Here's how the part is built. I have some questions about the finished solid (model axes, mm). A direction names the side the tool comes from. Give positions to 0.01 mm unless a question says otherwise; leave off trailing zeros. Write each loop counter-clockwise with the first axis right and the second up, starting at its lowest first coordinate (ties: lowest second). Pieces come first, ordered by that corner, then holes. Notation, with made-up numbers: (67.5, 85) - (79.5, 85) arc R17 cw to (79.5, 103) - close; hole circle Ø8 at (35.5, -38). An arc over 180 degrees is marked (long way). One line per item, written item: value. Start each with the question number.
1) Please list where these lines run through material, in increasing order: L1, parallel to X at y = 5, z = 0; L2, parallel to X at y = 14.5, z = -3; L3, parallel to Y at x = 2, z = 0. Write a range as [from, to].
2) Imagine slicing it at A-A on z = 0. Write out the boundary of the cut face in (x, y), plus the area to 3 significant figures.
3) We'd pull the mould along X, two halves only. Please class faces 1 (the flat face through (1, 4.5, 4.4)), 2 (the conical face through (0.51, -14.79, -10.76)), 3 (the conical face through (0.507, 1.163, -18.25)), 4 (the flat face through (0.014, 16.632, -0.983)): +X half, -X half, draft (parallel to the pull), parting line (faces both ways), or undercut.
4) I'm going to push flat-ended pins straight in: P1, Ø5, axis at x = 4, z = 6, coming from the +Y side; P2, Ø0.6, axis at x = 0, z = 0.5, coming from the -Y side; P3, Ø5, axis at x = 9, y = 5.5, coming from the +Z side. Where does each tip first touch, or does it pass through?
5) On a 3-axis mill with a long thin cutter (end or side, diameter ignored), from which of +Z, -Z, +X, -X, +Y, -Y can I reach the whole of each face in a straight line? I mean faces 5 (the conical face through (0.51, -3.41, -17.97)), 6 (the conical face through (-0.493, 13.331, -12.498)), 7 (the flat face through (0.01, 2.02, -16.49)). Say none if no direction works.
6) Imagine slicing it at C-C on x = 5.5. Write out the boundary of the cut face in (y, z), plus the area to 3 significant figures.
7) Imagine slicing it at B-B on x = 2.25. Write out the boundary of the cut face in (y, z), plus the area to 3 significant figures.
from build123d import *

# Parameters (mm, degrees)
SKETCH2_R           = 18.78
SKETCH2_R_2         = 4.05
BOSS_EXTRUDE1_DEPTH = 1
SKETCH9_R           = 6.05
SKETCH9_R_2         = 4.05
BOSS_EXTRUDE2_DEPTH = 10
SKETCH10_R          = 1.25
CUT_EXTRUDE1_DEPTH  = 10
CUT_EXTRUDE3_DEPTH  = 10
CIRPATTERN1_COUNT   = 25


with BuildPart() as part:
    # Sketch2 → Boss-Extrude1 (new, symmetric)
    with BuildSketch(Plane(origin=(0, 0, 0), x_dir=(0, 0, -1), z_dir=(1, 0, 0))):
        Circle(SKETCH2_R)
        Circle(SKETCH2_R_2, mode=Mode.SUBTRACT)
    extrude(amount=BOSS_EXTRUDE1_DEPTH, both=True)

    # Sketch9 → Boss-Extrude2 (add)
    with BuildSketch(Plane(origin=(1, 0, 0), x_dir=(0, 0, -1), z_dir=(1, 0, 0))):
        Circle(SKETCH9_R)
        Circle(SKETCH9_R_2, mode=Mode.SUBTRACT)
    extrude(amount=BOSS_EXTRUDE2_DEPTH)

    # Sketch5 → Cut-Revolve1 (revolve, cut)
    with BuildSketch(Plane(origin=(0, 0, 0), x_dir=(1, 0, 0), z_dir=(0, 1, 0)), mode=Mode.PRIVATE) as cut_revolve1_sk:
        Polygon((-1, -18.78), (0, -17.78), (1, -18.78), align=None)
    revolve(cut_revolve1_sk.sketch.rotate(Axis((11, 0, 0), (-1, 0, 0)), 180), axis=Axis((11, 0, 0), (-1, 0, 0)), mode=Mode.SUBTRACT)

    # Sketch10 → Cut-Extrude1 (cut, symmetric)
    with BuildSketch(Plane(origin=(0, 0, 0), x_dir=(1, 0, 0), z_dir=(0, 1, 0))):
        with Locations(Location((6, 0, 0), (0, 0, 270))):
            Circle(SKETCH10_R)
    extrude(amount=CUT_EXTRUDE1_DEPTH, both=True, mode=Mode.SUBTRACT)

    # Sketch12 → Cut-Extrude3 (cut, symmetric)
    with BuildSketch(Plane(origin=(1, 0, 0), x_dir=(0, 0, -1), z_dir=(1, 0, 0))):
        with BuildLine():
            ThreePointArc((-1.25, -18.738353716), (0, -18.78), (1.25, -18.738353716))
            Line((1.25, -18.738353716), (1.016521645, -15.238353716))
            Line((1.016521645, -15.238353716), (-1.016521645, -15.238353716))
            Line((-1.016521645, -15.238353716), (-1.25, -18.738353716))
        make_face()
    cut_extrude3 = extrude(amount=CUT_EXTRUDE3_DEPTH, both=True, mode=Mode.SUBTRACT)

    # CirPattern1: Cut-Extrude3 ×25 about axis
    cirpattern1_axis = Axis((0, 0, 0), (1, 0, 0))
    for i in range(1, CIRPATTERN1_COUNT):
        add(cut_extrude3.rotate(cirpattern1_axis, i * 360 / CIRPATTERN1_COUNT), mode=Mode.SUBTRACT)


solid = part.part
Numbers:
1. L1: [-1, 4.75], [7.25, 11]
1. L2: [-1, 1]
1. L3: [-6.05, -4.05], [4.05, 6.05]
2. outline: (-1, -15.24) - (1, -15.24) - (1, -6.05) - (4.75, -6.05) - (4.75, -4.05) - (-1, -4.05) - close; (-1, 4.05) - (4.75, 4.05) - (4.75, 6.05) - (1, 6.05) - (1, 18.78) - (0, 17.78) - (-1, 18.78) - close; (7.25, -6.05) - (11, -6.05) - (11, -4.05) - (7.25, -4.05) - close; (7.25, 4.05) - (11, 4.05) - (11, 6.05) - (7.25, 6.05) - close
2. area: 80.8 mm^2
3. face 1: +X half
3. face 2: undercut
3. face 3: undercut
3. face 4: draft
4. P1: y = 4.93
4. P2: y = -15.24
4. P3: z = 5.25
5. face 5: -Z, -Y
5. face 6: -Z, +Y
5. face 7: +X, -X
6. outline: (-5.94, -1.15) arc R6.05 ccw to (5.94, -1.15) - (3.88, -1.15) arc R4.05 cw to (-3.88, -1.15) - close; (-5.94, 1.15) - (-3.88, 1.15) arc R4.05 cw to (3.88, 1.15) - (5.94, 1.15) arc R6.05 ccw to start
6. area: 54.2 mm^2
7. outline: circle Ø12.1 at (0, 0); hole circle Ø8.1 at (0, 0)
7. area: 63.5 mm^2
